Here's how the part is built. I have some questions about the finished solid (model axes, mm). A direction names the side the tool comes from. Give positions to 0.01 mm unless a question says otherwise; leave off trailing zeros. Loops run counter-clockwise (first coordinate to the right, second up) from the corner with the lowest first, then second, coordinate; pieces in that order, holes last. Notation, with made-up numbers: M -27,24.25 L 3,24.25 A13 ccw 3,35.25 Z; hole C 34,84.25 d8. An arc over 180 degrees is marked long. Answer as CSV lines item,"result". Start each with the question number.
Item 1: For faces 4 (the flat face through (107.95, 89, 2)), 5 (the flat face through (69, 55, 3.175)), which set-ups out of +Z, -Z, +X, -X, +Y, -Y let a thin tool reach every point of the face, with its end or its side?
Item 2: I want a section at A-A on x = 54. List the corners of the cut face in (y, z) for me (3 decimals), plus the area to 3 significant figures.
Item 3: If we mould it in two halves opening along Y, with no side actions, what happens to faces 1 (the flat face through (44, 101.6, 2)), 2 (the flat face through (139.7, 69, 2)), 3 (the flat face through (69, 139.7, 2))? For each: released by +Y, released by -Y, zero draft, split by the parting line, or undercut.
Item 4: I want a section at B-B on y = 79. List the corners of the cut face in (x, z) for me (3 decimals), plus the area to 3 significant figures.
Item 5: If I drill on line 1 along Y through (x, z) = (70, 2.65); line 2 along Y through (x, z) = (52, 2.4); line 3 along X through (y, z) = (78, 2.9), over which ranges is the centre line in solid material (lowest first)? Write a range as from..to.
from build123d import *

# Parameters (mm, degrees)
SKETCH1_W           = 139.7
SKETCH1_H           = 139.7
BOSS_EXTRUDE1_DEPTH = 3.175


with BuildPart() as part:
    # Sketch1 → Boss-Extrude1 (new body)
    with BuildSketch(Plane.XY):
        with Locations((69.85, 69.85)):
            Rectangle(SKETCH1_W, SKETCH1_H)
        with BuildLine():
            Line((31.75, 101.6), (57.114301478, 101.6))
            add(Edge.make_bspline(
                [(57.114301478, 101.6), (69.85, 127), (82.585698522, 101.6)],
                knots=[0, 0, 0, 1, 1, 1], degree=2))
            Line((82.585698522, 101.6), (107.95, 101.6))
            Line((107.95, 101.6), (107.95, 76.2))
            Line((107.95, 76.2), (82.585698522, 76.2))
            add(Edge.make_bspline(
                [(57.114301478, 76.2), (69.85, 50.917743629), (82.585698522, 76.2)],
                knots=[0, 0, 0, 1, 1, 1], degree=2))
            Line((57.114301478, 76.2), (31.75, 76.2))
            Line((31.75, 76.2), (31.75, 101.6))
        make_face(mode=Mode.SUBTRACT)
    extrude(amount=BOSS_EXTRUDE1_DEPTH)


solid = part.part
Result:
1,face 4,"+Z, -Z"
1,face 5,"+Z, +X, -X, +Y, -Y"
2,outline,"M 0,0 L 76.2,0 L 76.2,3.175 L 0,3.175 Z; M 101.6,0 L 139.7,0 L 139.7,3.175 L 101.6,3.175 Z"
2,area,"363 mm^2"
3,face 1,"undercut"
3,face 2,"zero draft"
3,face 3,"released by +Y"
4,outline,"M 0,0 L 31.75,0 L 31.75,3.175 L 0,3.175 Z; M 107.95,0 L 139.7,0 L 139.7,3.175 L 107.95,3.175 Z"
4,area,"202 mm^2"
5,line 1,"0..63.56, 114.3..139.7"
5,line 2,"0..76.2, 101.6..139.7"
5,line 3,"0..31.75, 107.95..139.7"
